The model under review builds one solid part; all positions refer to its coordinate system, in mm. Face numbers are marked on the shaded views. A direction names the side the tool comes from. Coordinates: 2 decimals unless noted, no trailing zeros. Order: outer loops, then holes, each group sorted by start corner. A loop starts at its lowest first (then second) coordinate and runs counter-clockwise, first axis right, second up. Notation, with made-up numbers: (18.5, 62) -> (48.5, 62) arc R19 cw to (48.5, 75) -> close; hole circle Ø5 at (-0.5, 25.5). An arc over 180 degrees is marked (long way). Use one line per item in the form item = value.
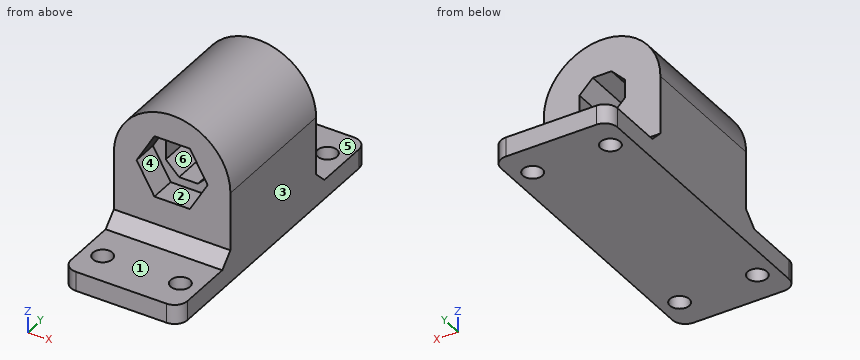
from build123d import *

# Parameters (mm, degrees)
BOSS_EXTRUDE1_DEPTH = 21
BOSS_EXTRUDE2_START = -17
SKETCH2_R           = 9
BOSS_EXTRUDE2_DEPTH = 17
SKETCH4_W           = 18
SKETCH4_H           = 12.5
SKETCH4_R           = 1.5
BOSS_EXTRUDE3_DEPTH = 3
FILLET1_R           = 2
CHAMFER1_SIZE       = 2


with BuildPart() as part:
    # Sketch1 → Boss-Extrude1 (new body)
    with BuildSketch(Plane(origin=(0, 0, 0), x_dir=(1, 0, 0), z_dir=(0, 1, 0))):
        with BuildLine():
            Line((-9, 0), (9, 0))
            Line((9, 0), (9, -14))
            ThreePointArc((9, -14), (0, -23), (-9, -14))
            Line((-9, -14), (-9, 0))
        make_face()
        Polygon((-2.742413779, -9.25), (-5.484827557, -14), (-2.742413779, -18.75), (2.742413779, -18.75), (5.484827557, -14), (2.742413779, -9.25), align=None, mode=Mode.SUBTRACT)
    extrude(amount=BOSS_EXTRUDE1_DEPTH)

    # Sketch2 → Boss-Extrude2 (add)
    with BuildSketch(Plane(origin=(0, 21, 0), x_dir=(1, 0, 0), z_dir=(0, 1, 0)).offset(BOSS_EXTRUDE2_START)):
        with Locations((0, -14)):
            Circle(SKETCH2_R)
        Polygon((3.5, -12.550252532), (1.449747468, -10.5), (-1.449747468, -10.5), (-3.5, -12.550252532), (-3.5, -15.449747468), (-1.449747468, -17.5), (1.449747468, -17.5), (3.5, -15.449747468), align=None, mode=Mode.SUBTRACT)
    extrude(amount=BOSS_EXTRUDE2_DEPTH)

    # Sketch4 → Boss-Extrude3 (add)
    # profile 1 of 2: a face of its own
    with BuildSketch(Plane(origin=(0, 0, 0), x_dir=(-1, 0, 0), z_dir=(0, 0, -1))):
        with Locations((0, 27.25)):
            Rectangle(SKETCH4_W, SKETCH4_H)
        with Locations((-6, 28.5)):
            Circle(SKETCH4_R, mode=Mode.SUBTRACT)
        with Locations((6, 28.5)):
            Circle(SKETCH4_R, mode=Mode.SUBTRACT)
    # profile 2 of 2: a face of its own
    with BuildSketch(Plane(origin=(0, 0, 0), x_dir=(-1, 0, 0), z_dir=(0, 0, -1))):
        with Locations((0, -6.25)):
            Rectangle(SKETCH4_W, SKETCH4_H)
        with Locations(Location((6, -7.5, 0), (0, 0, 180))):
            Circle(SKETCH4_R, mode=Mode.SUBTRACT)
        with Locations(Location((-6, -7.5, 0), (0, 0, 180))):
            Circle(SKETCH4_R, mode=Mode.SUBTRACT)
    extrude(amount=-BOSS_EXTRUDE3_DEPTH)

    # Fillet1
    fillet1_edges = [part.edges().sort_by_distance(p)[0] for p in [
        (9, 33.5, 1.5),
        (-9, 33.5, 1.5),
        (-9, -12.5, 1.5),
        (9, -12.5, 1.5),
    ]]
    fillet(fillet1_edges, radius=FILLET1_R)

    # Chamfer1
    chamfer1_edges = [part.edges().sort_by_distance(p)[0] for p in [
        (0, 21, 3),
        (0, 0, 3),
    ]]
    chamfer(chamfer1_edges, length=CHAMFER1_SIZE)


solid = part.part
Item 1: We need section B-B (y = -7.5). Write out the cut boundary in (x, z), plus the area to 3 significant figures.
Results found:
outline = (-9, 0) -> (-7.5, 0) -> (-7.5, 3) -> (-9, 3) -> close; (-4.5, 0) -> (4.5, 0) -> (4.5, 3) -> (-4.5, 3) -> close; (7.5, 0) -> (9, 0) -> (9, 3) -> (7.5, 3) -> close
area = 36.0 mm²
Item 2: Clearance check with flat-ended pins moving along their axes: pin 1 (5.5 mm diameter, centred on x = 0.5, z = 13, fed in from -Y); pin 2 (10 mm diameter, centred on x = -2, z = 17, fed in from -Y); pin 3 (1.5 mm diameter, centred on x = 5.5, z = 4, fed in from -Y). State where each tip first meets the part, or that it passes through.
Results found:
pin_1 = 4
pin_2 = 0
pin_3 = -1.75
Item 3: We need section D-D (x = -6). Write out the cut boundary in (y, z).
Results found:
outline = (-12.5, 0) -> (-9, 0) -> (-9, 3) -> (-12.5, 3) -> close; (-6, 0) -> (27, 0) -> (27, 3) -> (23, 3) -> (21, 5) -> (21, 20.71) -> (0, 20.71) -> (0, 5) -> (-2, 3) -> (-6, 3) -> close; (30, 0) -> (33.5, 0) -> (33.5, 3) -> (30, 3) -> close
Item 4: Draft analysis for pull direction Z (two halves, no side actions). For the marked faces 1, 2 and 3, state which applies: released by +Z, released by -Z, zero draft, split by the parting line, or undercut.
Results found:
face_1 = released by +Z
face_2 = undercut
face_3 = zero draft
Item 5: Tool access review of the marked faces 4, 5 and 6: name each direction out of +Z, -Z, +X, -X, +Y, -Y from which nothing blocks a thin tool from reaching the whole face with its end or side.
Results found:
face_4 = -Y
face_5 = +Z, +X, -X, +Y
face_6 = +Y, -Y
Item 6: To check wall thickness, follow L1, parallel to Y at x = -6, z = 1.95; L2, parallel to X at y = -7.5, z = 2.4; L3, parallel to Y at x = -3.5, z = 18. State the ranges of each line that lie inside material, in increasing order. Write a range as from..to.
Results found:
L1 = -12.5..-9, -6..27, 30..33.5
L2 = -9..-7.5, -4.5..4.5, 7.5..9
L3 = 0..21
Item 7: We need section A-A (x = 0). Write out the cut boundary in (y, z), plus the area to 3 significant figures.
Results found:
outline = (-12.5, 0) -> (33.5, 0) -> (33.5, 3) -> (23, 3) -> (21, 5) -> (21, 10.5) -> (4, 10.5) -> (4, 9.25) -> (0, 9.25) -> (0, 5) -> (-2, 3) -> (-12.5, 3) -> close; (0, 18.75) -> (4, 18.75) -> (4, 17.5) -> (21, 17.5) -> (21, 23) -> (0, 23) -> close
area = 405 mm²
Item 8: We need section C-C (y = 14). Write out the cut boundary in (x, z).
Results found:
outline = (-9, 0) -> (9, 0) -> (9, 14) arc R9 ccw to (-9, 14) -> close; hole (-3.5, 12.55) -> (-1.45, 10.5) -> (1.45, 10.5) -> (3.5, 12.55) -> (3.5, 15.45) -> (1.45, 17.5) -> (-1.45, 17.5) -> (-3.5, 15.45) -> close
